from build123d import *

# Parameters (mm, degrees)
BASE_FLANGE1_DEPTH          = 111.125
CUT_EXTRUDE1_REACH          = 143.492
F_1_4_20_TAPPED_HOLE1_D     = 5.1054
EXTRUDE1_REACH              = 143.492
SKETCH5_W                   = 120.65
SKETCH5_H                   = 22.225
FILLET2_R                   = 12.7
F_1_4_20_TAPPED_HOLE2_D     = 5.1054
F_1_4_20_TAPPED_HOLE2_DEPTH = 16.51
F_1_4_20_TAPPED_HOLE2_TIP   = 1.533816902
SKETCH8_W                   = 63.5
SKETCH8_H                   = 34.925
CUT_EXTRUDE2_DEPTH          = 12.7
CHAMFER1_SIZE               = 15.875
FILLET3_R                   = 9.525
FILLET4_R                   = 9.525
FILLET5_R                   = 6.35


# Sheet-metal steps are written as plain solids
with BuildPart() as part:
    # Sketch1 → Base-Flange1 (new, symmetric)
    with BuildSketch(Plane.XY):
        with BuildLine():
            Line((0, 60.325), (0, 6.35))
            ThreePointArc((0, 6.35), (1.859871939, 1.859871939), (6.35, 0))
            Line((6.35, 0), (63.5, 0))
            Line((63.5, 0), (63.5, 3.175))
            Line((63.5, 3.175), (6.35, 3.175))
            ThreePointArc((6.35, 3.175), (4.10493597, 4.10493597), (3.175, 6.35))
            Line((3.175, 6.35), (3.175, 60.325))
            Line((3.175, 60.325), (0, 60.325))
        make_face()
    extrude(amount=BASE_FLANGE1_DEPTH, both=True)

    # Sketch2 → Cut-Extrude1 (cut, up to next)
    with BuildSketch(Plane.XZ, mode=Mode.PRIVATE) as cut_extrude1_sk1:
        with BuildLine():
            Line((31.75, 60.721875), (57.15, 60.721875))
            ThreePointArc((57.15, 60.721875), (60.721875, 57.15), (57.15, 53.578125))
            Line((57.15, 53.578125), (31.75, 53.578125))
            ThreePointArc((31.75, 53.578125), (28.178125, 57.15), (31.75, 60.721875))
        make_face()
    cut_extrude1_tool1 = extrude(cut_extrude1_sk1.sketch, amount=-CUT_EXTRUDE1_REACH, mode=Mode.PRIVATE) & part.part
    # Sketch2 → Cut-Extrude1 (cut, up to next)
    with BuildSketch(Plane.XZ, mode=Mode.PRIVATE) as cut_extrude1_sk2:
        with BuildLine():
            Line((31.75, -53.578125), (57.15, -53.578125))
            ThreePointArc((57.15, -53.578125), (60.721875, -57.15), (57.15, -60.721875))
            Line((57.15, -60.721875), (31.75, -60.721875))
            ThreePointArc((31.75, -60.721875), (28.178125, -57.15), (31.75, -53.578125))
        make_face()
    cut_extrude1_tool2 = extrude(cut_extrude1_sk2.sketch, amount=-CUT_EXTRUDE1_REACH, mode=Mode.PRIVATE) & part.part
    add(cut_extrude1_tool1.solids().sort_by_distance((44.45, 0, 57.15))[0], mode=Mode.SUBTRACT)
    add(cut_extrude1_tool2.solids().sort_by_distance((44.45, 0, -57.15))[0], mode=Mode.SUBTRACT)

    # 1/4-20 Tapped Hole1 (through all)
    with Locations(Plane.ZY):
        with Locations((-92.075, 31.75), (92.075, 31.75)):
            Hole(F_1_4_20_TAPPED_HOLE1_D / 2)

    # Sketch5 → Extrude1 (cut, up to next)
    with BuildSketch(Plane.ZY, mode=Mode.PRIVATE) as extrude1_sk1:
        with Locations((0, 49.2125)):
            Rectangle(SKETCH5_W, SKETCH5_H)
    extrude1_tool1 = extrude(extrude1_sk1.sketch, amount=-EXTRUDE1_REACH, mode=Mode.PRIVATE) & part.part
    add(extrude1_tool1.solids().sort_by_distance((0, 49.2125, 0))[0], mode=Mode.SUBTRACT)

    # Fillet2
    fillet2_edges = [part.edges().sort_by_distance(p)[0] for p in [
        (1.5875, 38.1, -60.325),
        (1.5875, 38.1, 60.325),
    ]]
    fillet(fillet2_edges, radius=FILLET2_R)

    # 1/4-20 Tapped Hole2
    with Locations(Plane(origin=(3.175, 0, 0), x_dir=(0, 0, -1), z_dir=(1, 0, 0))):
        with Locations((-50.8, 25.4), (50.8, 25.4)):
            Hole(F_1_4_20_TAPPED_HOLE2_D / 2, depth=F_1_4_20_TAPPED_HOLE2_DEPTH)
            with Locations((0, 0, -(F_1_4_20_TAPPED_HOLE2_DEPTH + F_1_4_20_TAPPED_HOLE2_TIP / 2))):  # 118° drill point
                Cone(0, F_1_4_20_TAPPED_HOLE2_D / 2, F_1_4_20_TAPPED_HOLE2_TIP, mode=Mode.SUBTRACT)

    # Sketch8 → Cut-Extrude2 (cut)
    with BuildSketch(Plane.XZ):
        with Locations((31.75, 93.6625)):
            Rectangle(SKETCH8_W, SKETCH8_H)
        with Locations((31.75, -93.6625)):
            Rectangle(SKETCH8_W, SKETCH8_H)
    extrude(amount=-CUT_EXTRUDE2_DEPTH, mode=Mode.SUBTRACT)

    # Chamfer1
    chamfer1_edges = [part.edges().sort_by_distance(p)[0] for p in [
        (1.5875, 12.7, 111.125),
        (1.5875, 12.7, -111.125),
    ]]
    chamfer(chamfer1_edges, length=CHAMFER1_SIZE)

    # Fillet3
    fillet3_edges = [part.edges().sort_by_distance(p)[0] for p in [
        (1.5875, 60.325, -111.125),
        (1.5875, 60.325, -60.325),
        (1.5875, 60.325, 60.325),
        (1.5875, 60.325, 111.125),
        (63.5, 1.5875, -76.2),
        (63.5, 1.5875, 76.2),
    ]]
    fillet(fillet3_edges, radius=FILLET3_R - 0.0001)  # a hair under: the kernel refuses the full size

    # Fillet4
    fillet4_edges = [part.edges().sort_by_distance(p)[0] for p in [
        (1.5875, 12.7, 95.25),
        (1.5875, 28.575, 111.125),
        (1.5875, 12.7, -95.25),
        (1.5875, 28.575, -111.125),
    ]]
    fillet(fillet4_edges, radius=FILLET4_R)

    # Fillet5
    fillet5_edges = [part.edges().sort_by_distance(p)[0] for p in [
        (1.5875, 12.7, -76.2),
        (1.5875, 12.7, 76.2),
    ]]
    fillet(fillet5_edges, radius=FILLET5_R)


solid = part.part
CAD build for the part. Positions are in the model's coordinates, mm. A direction names the side the tool comes from. Coordinates: 2 decimals unless noted, no trailing zeros. Write each loop counter-clockwise with the first axis right and the second up, starting at its lowest first coordinate (ties: lowest second). Pieces come first, ordered by that corner, then holes. Notation, with made-up numbers: (78.5, -22) - (128.5, -22) arc R7 cw to (128.5, -16) - close; hole circle Ø11 at (63.5, -28.75). An arc over 180 degrees is marked (long way). Use a Markdown table: item, result. Add a question column.
Item 1: Band-saw the part on D-D, the plane x = 11. Give the cut face in (y, z) (3 decimals).
Item 2: Band-saw the part on C-C, the plane z = 13.5. Give the cut face in (x, y) (3 decimals), and give its area (3 significant figures).
Item 3: Flat gauge pins, fed straight in: pin 1 (1.6 mm diameter, centred on x = 1.5, z = 88, fed in from -Y); pin 2 (7 mm diameter, centred on x = 18, y = 4, fed in from -Z); pin 3 (8 mm diameter, centred on y = 31.5, z = -84.5, fed in from +X) (3 decimals). Where does each tip first touch, or does it go through?
Item 4: 3-axis set-ups, long thin cutter, end or side, ignore diameter. For faces 1 (the face through (35, 3.175, 1)), 2 (the face through (1.61, 57.46, -63.04)), 3 (the face through (27, 2, 76.2)), 4 (the face through (27, 2, -76.2)): which of +Z, -Z, +X, -X, +Y, -Y reach the whole face in a straight line?
Item 5: Mould opens along Z. For faces 5 (the face through (1.57, 20.71, -103.26)), 6 (the face through (1.57, 57.46, 108.41)), 7 (the face through (1.61, 41.722, 56.506)) say: pulls with the +Z half, pulls with the -Z half, needs draft (parallel to the pull), parting line crosses it, or undercut.
Item 6: Drill centre lines: L1, parallel to Z at x = 2, y = 31; L2, parallel to Y at x = 24, z = 47 (3 decimals). Where is each one in solid material? Low to high. Write a range as from..to.
Item 7: Band-saw the part on B-B, the plane z = 57.15. Give the cut face in (x, y) (3 decimals).
Item 8: Band-saw the part on A-A, the plane y = 48. Give the cut face in (x, z) (1 decimal), and give its area (3 significant figures).
Numbers:
| question | item | result |
|---|---|---|
| 1 | outline | (0, -76.2) - (3.175, -76.2) - (3.175, 76.2) - (0, 76.2) - close |
| 2 | outline | (0, 6.35) arc R6.35 ccw to (6.35, 0) - (63.5, 0) - (63.5, 3.175) - (6.35, 3.175) arc R3.175 cw to (3.175, 6.35) - (3.175, 38.1) - (0, 38.1) - close |
| 2 | area | 306 mm2 |
| 3 | pin 1 | y = 12.7 |
| 3 | pin 2 | z = -76.2 |
| 3 | pin 3 | x = 3.175 |
| 4 | face 1 | +Z, -Z, +X, +Y |
| 4 | face 2 | +X, -X, +Y |
| 4 | face 3 | +Z, +X, -X, -Y |
| 4 | face 4 | -Z, +X, -X, -Y |
| 5 | face 5 | pulls with the -Z half |
| 5 | face 6 | pulls with the +Z half |
| 5 | face 7 | undercut |
| 6 | L1 | -111..-94.52, -89.63..89.63, 94.52..111 |
| 6 | L2 | 0..3.175 |
| 7 | outline | (0, 6.35) arc R6.35 ccw to (6.35, 0) - (28.178, 0) - (28.178, 3.175) - (6.35, 3.175) arc R3.175 cw to (3.175, 6.35) - (3.175, 42.4) - (0, 42.4) - close; (60.722, 0) - (63.5, 0) - (63.5, 3.175) - (60.722, 3.175) - close |
| 8 | outline | (0, -111.1) - (3.2, -111.1) - (3.2, -60) - (0, -60) - close; (0, 60) - (3.2, 60) - (3.2, 111.1) - (0, 111.1) - close |
| 8 | area | 325 mm2 |
